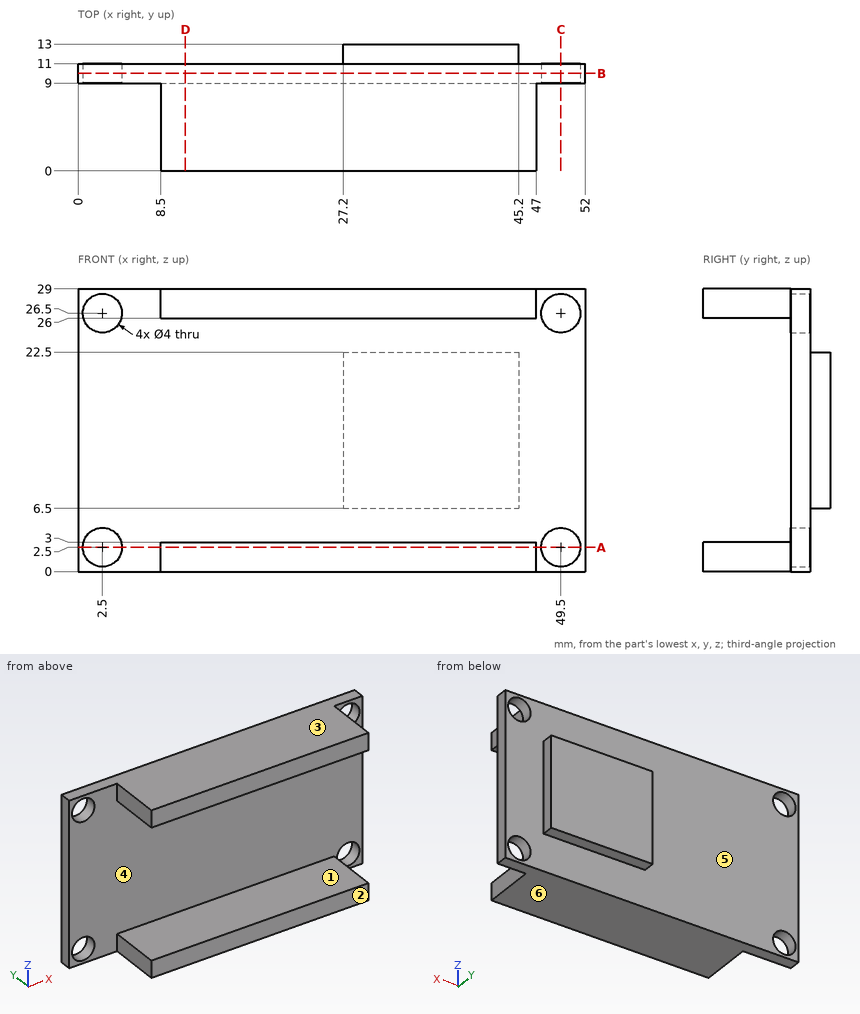
Check sheet for the drawn part. Datum: minimum x, y, z corner. Units: mm. A direction names the side the tool comes from. Coordinates: 2 decimals unless noted, no trailing zeros. Loops run counter-clockwise (first coordinate to the right, second up) from the corner with the lowest first, then second, coordinate; pieces in that order, holes last. Notation, with made-up numbers: M -29.5,65.5 L 4.5,65.5 A6 ccw 4.5,74.5 Z; hole C 7.5,49.25 d4. An arc over 180 degrees is marked long. Answer as a JSON object with one key per item and string values.
1. Sectioned sample at C-C on x = 49.5. Record the cut outline in (y, z), and give its area (3 significant figures).
Outcome:
{"outline": "M 9,0 L 11,0 L 11,0.5 L 9,0.5 Z; M 9,4.5 L 11,4.5 L 11,24.5 L 9,24.5 Z; M 9,28.5 L 11,28.5 L 11,29 L 9,29 Z", "area": "42.0 mm²"}
2. Sectioned sample at B-B on y = 10. Record the cut outline in (x, z).
Outcome:
{"outline": "M 0,0 L 52,0 L 52,29 L 0,29 Z; hole C 2.5,2.5 d4; hole C 2.5,26.5 d4; hole C 49.5,2.5 d4; hole C 49.5,26.5 d4"}
3. Release check for a two-part mould opening along Z. For the marked faces 3, 4, 5 and 6 record: pulls with the +Z half, pulls with the -Z half, needs draft (parallel to the pull), parting line crosses it, or undercut.
Outcome:
{"face 3": "pulls with the +Z half", "face 4": "undercut", "face 5": "needs draft", "face 6": "pulls with the -Z half"}
4. Access from +Z, -Z, +X, -X, +Y, -Y to the whole of each face (thin tool, end or side, straight path). Record for the marked faces 1 and 2.
Outcome:
{"face 1": "+X, -X, -Y", "face 2": "+Z, -Z, +X, -X, -Y"}
5. Sectioned sample at D-D on x = 11. Record the cut outline in (y, z).
Outcome:
{"outline": "M 0,0 L 11,0 L 11,29 L 0,29 L 0,26 L 9,26 L 9,3 L 0,3 Z"}
6. Sectioned sample at A-A on z = 2.5. Record the cut outline in (x, y).
Outcome:
{"outline": "M 0,9 L 0.5,9 L 0.5,11 L 0,11 Z; M 4.5,9 L 8.5,9 L 8.5,0 L 47,0 L 47,9 L 47.5,9 L 47.5,11 L 4.5,11 Z; M 51.5,9 L 52,9 L 52,11 L 51.5,11 Z"}
7. Scan lines: L1, parallel to X at y = 9.8, z = 2.5; L2, parallel to Z at x = 24, y = 6.75; L3, parallel to Y at x = 18.5, z = 9. Record each from-to range of solid material in increasing order. Write a range as from..to.
Outcome:
{"L1": "0..0.5, 4.5..47.5, 51.5..52", "L2": "0..3, 26..29", "L3": "9..11"}
8. Depth check by flat-ended pin: P1, Ø0.9, axis at y = 2.5, z = 1.5, coming from the -X side; P2, Ø3.5, axis at y = 6.5, z = 2, coming from the +X side; P3, Ø8.5, axis at x = 20, z = 18, coming from the -Y side; P4, Ø1, axis at x = 7, y = 5, coming from the +Z side. Enter the tip coordinate at first touch or a pass-through.
Outcome:
{"P1": "x = 8.5", "P2": "x = 47", "P3": "y = 9", "P4": "through"}
